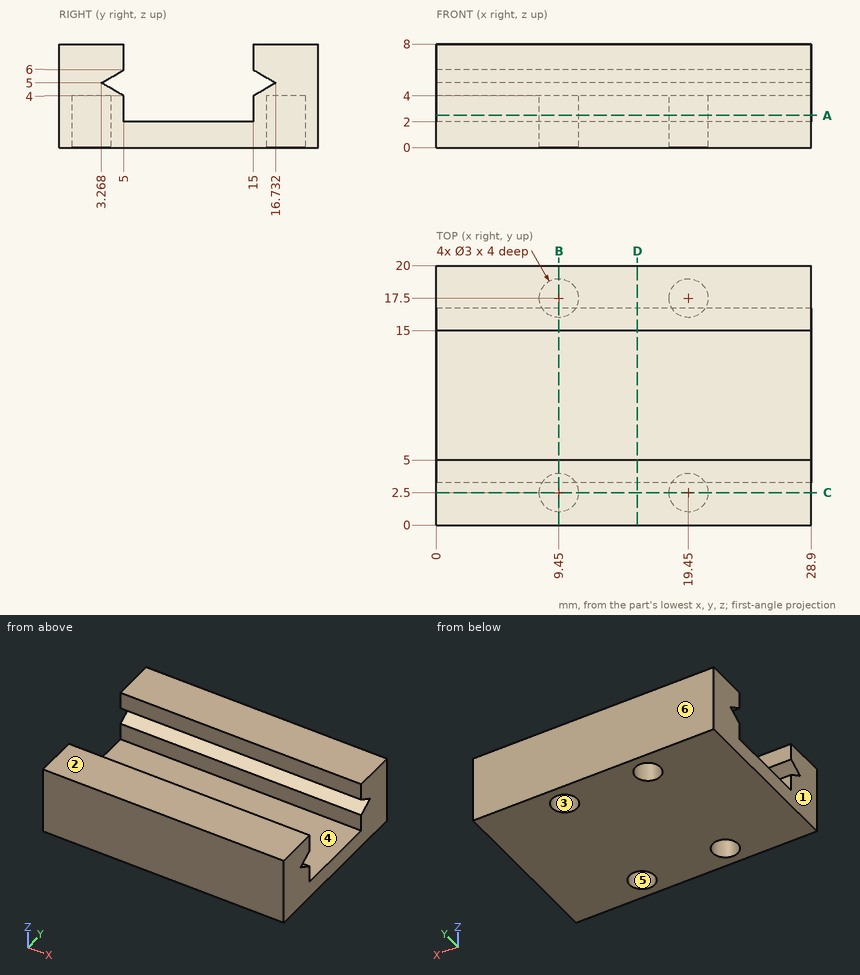
Study the drawing (mm; zero at the part's minimum x, y, z) and answer. A direction names the side the tool comes from. Give positions to 0.01 mm unless a question says otherwise; leave off trailing zeros. Order: outer loops, then holes, each group sorted by start corner. A loop starts at its lowest first (then second) coordinate and runs counter-clockwise, first axis right, second up.
1. Section D-D, the plane x = 15.5 is taken. Determine the outline of the cut face in (y, z).
Result sheet:
outline: (0, 0) - (20, 0) - (20, 8) - (15, 8) - (15, 6) - (16.73, 5) - (15, 4) - (15, 2) - (5, 2) - (5, 4) - (3.27, 5) - (5, 6) - (5, 8) - (0, 8) - close
2. Section A-A, the plane z = 2.5 is taken. Determine the outline of the cut face in (x, y).
Result sheet:
outline: (0, 0) - (28.9, 0) - (28.9, 5) - (0, 5) - close; (0, 15) - (28.9, 15) - (28.9, 20) - (0, 20) - close; hole circle Ø3 at (9.45, 2.5); hole circle Ø3 at (9.45, 17.5); hole circle Ø3 at (19.45, 2.5); hole circle Ø3 at (19.45, 17.5)
3. Each of these flat-tipped pins is pushed along its axis until it touches: P1, Ø0.9, axis at x = 19, y = 18, coming from the -Z side; P2, Ø6, axis at x = 22.5, y = 10, coming from the +Z side. Where does it stop, or does it pass through?
Result sheet:
P1: stops at z = 4
P2: stops at z = 2
4. Section B-B, the plane x = 9.45 is taken. Determine the outline of the cut face in (y, z).
Result sheet:
outline: (0, 0) - (1, 0) - (1, 4) - (4, 4) - (4, 0) - (16, 0) - (16, 4) - (19, 4) - (19, 0) - (20, 0) - (20, 8) - (15, 8) - (15, 6) - (16.73, 5) - (15, 4) - (15, 2) - (5, 2) - (5, 4) - (3.27, 5) - (5, 6) - (5, 8) - (0, 8) - close
5. For the marked faces 4, 5 and 6, determine the directions among +Z, -Z, +X, -X, +Y, -Y from which every point of the face is accessible in a straight line to the end or side of a thin tool.
Result sheet:
face 4: +Z, +X, -X
face 5: -Z
face 6: +Z, -Z, +X, -X, +Y
6. Straight lines are drawn through the part: L1, parallel to Y at x = 9.45, z = 2.95; L2, parallel to Y at x = 9.45, z = 0.95; L3, parallel to Y at x = 25.5, z = 6.75. For each, find the intervals that lie inside material, in ascending order.
Result sheet:
L1: y = 0 to 1, 4 to 5, 15 to 16, 19 to 20
L2: y = 0 to 1, 4 to 16, 19 to 20
L3: y = 0 to 5, 15 to 20
7. The mould has two halves that part along X. Classify the marked faces 1, 2 and 3: released by +X, released by -X, zero draft, split by the parting line, or undercut.
Result sheet:
face 1: released by -X
face 2: zero draft
face 3: undercut
8. Section C-C, the plane y = 2.5 is taken. Determine the outline of the cut face in (x, z).
Result sheet:
outline: (0, 0) - (7.95, 0) - (7.95, 4) - (10.95, 4) - (10.95, 0) - (17.95, 0) - (17.95, 4) - (20.95, 4) - (20.95, 0) - (28.9, 0) - (28.9, 8) - (0, 8) - close
